Autodesk Inventor part; units mm, degrees
ref_plane "Work Plane4" through (-13.97, 12.7, 0) normal (0, 1, 0) x (1, 0, 0)
ref_plane "Work Plane5" through (-3.3455, -30.0155, 0) normal (0, 1, 0) x (-1, 0, 0)
ref_plane "YZ Plane" through (0, 0, 0) normal (1, 0, 0) x (0, 1, 0)
sketch "Sketch1" plane through (0, 0, 0) normal (0, 0, 1) x (1, 0, 0)
  line L0 (-13.97, -12.7) -> (13.97, -12.7)
  line L1 (13.97, -12.7) -> (13.97, 12.7)
  line L2 (13.97, 12.7) -> (-13.97, 12.7)
  line L3 (-13.97, 12.7) -> (-13.97, -12.7)
  line L4 (-13.97, -12.7) -> (13.97, 12.7) construction
  line L5 (13.97, -12.7) -> (-13.97, 12.7) construction
  arc A0 (-13.97, -12.7) -> (13.97, -12.7) centre (0, -12.7) ccw
  circle A1 centre (-3.3455, -12.7) radius 11.811
  line L6 (0, -12.7) -> (-13.97, -12.7)
  line L7 (0, -12.7) -> (-6.985, -12.7)
  circle A2 centre (-3.3455, -12.7) radius 17.3155
  arc A3 (-20.6609, -12.7) -> (-13.97, 12.7) centre (-56.001, 10.1906) ccw
  point P0 (0, 0)
  point P1 (-15.1565, -0.038)
  dimension "d0" = 27.94
  dimension "d1" = 25.4
  dimension "d2" = 23.622
sketch "Sketch5" plane through (0, 0, 0) normal (0, 0, 1) x (1, 0, 0)
  line L0 (0, 12.7) -> (0, 6.35)
  line L1 (0, 12.7) -> (0, 9.525)
  line L2 (5.715, 7.3025) -> (-5.715, 7.3025)
  line L3 (-5.715, 7.3025) -> (-5.715, 11.7475)
  line L4 (-5.715, 11.7475) -> (5.715, 11.7475)
  line L5 (5.715, 11.7475) -> (5.715, 7.3025)
  line L6 (5.715, 7.3025) -> (-5.715, 11.7475) construction
  line L7 (-5.715, 7.3025) -> (5.715, 11.7475) construction
  line L8 (5.715, 11.7475) -> (3.175, 11.7475)
  line L9 (3.175, 11.7475) -> (3.175, 10.7597)
  line L10 (3.175, 10.7597) -> (5.715, 10.7597)
  line L11 (5.715, 10.7597) -> (5.715, 11.7475)
  line L12 (-5.715, 11.7475) -> (-3.2581, 11.7475)
  line L13 (-3.2581, 11.7475) -> (-3.2581, 10.792)
  line L14 (-3.2581, 10.792) -> (-5.715, 10.792)
  line L15 (-5.715, 10.792) -> (-5.715, 11.7475)
  line L16 (5.715, 9.525) -> (3.175, 7.3025)
  line L17 (-5.715, 9.525) -> (-3.175, 7.3025)
  point P0 (0, 0)
  point P1 (5.715, 10.7597)
  point P2 (-3.2581, 11.7475)
  point P3 (-5.715, 10.792)
  dimension "d5" = 4.445
  dimension "d6" = 11.43
  dimension "d7" = 2.54
ref_plane "Work Plane4" through (-13.97, 12.7, 0) normal (0, 1, 0) x (1, 0, 0)
sketch "Sketch6" plane through (-13.97, 12.7, 0) normal (0, 1, 0) x (1, 0, 0)
  circle A0 centre (13.5492, -9.5343) radius 2.54
  dimension "d19" = 5.08
extrude "Extrusion7" add sketch "Sketch1" along normal blind 19.05 contours A1 A0 A2 A3 L3 | L3 A2 L0 A1 | A1 L0 A0 | A2 A3 L3 | L3 A3 L2 L1 A2 | A3 A2 picked at (12.0052, -13.7923)
extrude "Extrusion8" cut sketch "Sketch5" along normal blind 20.32 contours L4 L9 L10 L5 L16 L2 L0 | L0 L2 L17 L3 L14 L13 L4
extrude "Extrusion9" cut sketch "Sketch6" against normal blind 15.24
fillet "Fillet1" radius 3.175 1 edges at (-15.1565, -0.038, 9.525)
sketch "Sketch10" plane through (-13.97, 12.7, 0) normal (0, 1, 0) x (1, 0, 0)
  line L0 (13.97, 0) -> (13.97, -20.32)
  line L1 (0.0748, -19.05) -> (0.0748, 0)
  line L2 (0.0748, -9.525) -> (27.94, -9.525)
  line L3 (27.94, 0) -> (27.94, -19.05)
  line L4 (3.9773, -13.335) -> (1.6913, -13.335)
  line L5 (1.6913, -13.335) -> (1.6913, -5.715)
  line L6 (1.6913, -5.715) -> (3.9773, -5.715)
  line L7 (3.9773, -5.715) -> (3.9773, -13.335)
  line L8 (3.9773, -13.335) -> (1.6913, -5.715) construction
  line L9 (1.6913, -13.335) -> (3.9773, -5.715) construction
  line L10 (23.9627, -13.335) -> (26.2487, -13.335)
  line L11 (26.2487, -13.335) -> (26.2487, -5.715)
  line L12 (26.2487, -5.715) -> (23.9627, -5.715)
  line L13 (23.9627, -5.715) -> (23.9627, -13.335)
  point P0 (2.8343, -9.525)
  dimension "d32" = 2.286
  dimension "d33" = 7.62
extrude "Extrusion10" cut sketch "Sketch10" against normal blind 2.54
ref_plane "Work Plane5" through (-3.3455, -30.0155, 0) normal (0, 1, 0) x (-1, 0, 0)
sketch "Sketch11" plane through (-3.3455, -30.0155, 0) normal (0, 1, 0) x (-1, 0, 0)
  line L0 (-0.1705, 0) -> (-0.1705, 19.05)
  circle A0 centre (-0.1705, 9.525) radius 2.54
  point P0 (-3.3455, 0)
  dimension "d36" = 5.08
extrude "Extrusion11" cut sketch "Sketch11" along normal blind 15.24
properties part number "MotorBearingHolder"
CAD build for the part. Positions are in the model's coordinates, mm. A direction names the side the tool comes from. Round coordinates to 2 decimals unless told otherwise and drop trailing zeros. Write each loop counter-clockwise with the first axis right and the second up, starting at its lowest first coordinate (ties: lowest second). Pieces come first, ordered by that corner, then holes.
(1) Slice it at D-D, the plane z = 14. Count the separate pieces of the cut face and the enclosed holes in it, and give its area (3 significant figures).
(2) Mould opens along Z. For faces 4 (the face through (9.993, 11, 9)), 5 (the face through (-14.03, 6.84, 9.39)), 6 (the face through (11, 11, 5.715)) say: pulls with the +Z half, pulls with the -Z half, needs draft (parallel to the pull), parting line crosses it, or undercut.
(3) Slice it at B-B, the plane x = -9.5. Write the cut outline in (y, z).
(4) Probe line 1 along Y through (x, z) = (5, 12.75); line 2 along Y through (x, z) = (2.5, 9.75); line 3 along X through (y, z) = (-12.7, 7.5). List the from-to ranges inside material, lowest first.
(5) Slice it at C-C, the plane x = -4. Write the cut outline in (y, z), and give its area (3 significant figures).
(6) Drop flat-ended pins along their axis: P1, Ø1.3, axis at y = 11.5, z = 11, coming from the -X side; P2, Ø2, axis at x = -6, y = -22, coming from the +Z side; P3, Ø1.8, axis at x = 11, z = 11, coming from the +Y side; P4, Ø3, axis at x = -0.5, z = 12, coming from the -Y side. Give the stop position or say it passes through.
(7) 3-axis set-ups, long thin cutter, end or side, ignore diameter. For faces 1 (the face through (-12.279, 11, 10)), 2 (the face through (-4, 10.792, 9)), 3 (the face through (13.97, 0, 9)): which of +Z, -Z, +X, -X, +Y, -Y reach the whole face in a straight line?
(8) Slice it at A-A, the plane y = -21. Write the cut outline in (x, z).
From the geometry:
1. separate pieces: 1
1. enclosed holes: 2
1. area: 769 mm2
2. face 4: undercut
2. face 5: needs draft
2. face 6: undercut
3. outline: (-28.88, 0) - (-22.78, 0) - (-22.78, 19.05) - (-28.88, 19.05) - close; (-2.62, 0) - (12.7, 0) - (12.7, 19.05) - (-2.62, 19.05) - close
4. line 1: y = -27.87 to -21.06, -4.34 to 8.9, 10.76 to 12.7
4. line 2: y = -29 to -22.96, -2.44 to 7.3, 11.75 to 12.7
4. line 3: x = -20.66 to -15.16, 8.47 to 13.97
5. outline: (-30, 0) - (-24.49, 0) - (-24.49, 7.12) - (-30, 7.12) - close; (-30, 11.93) - (-24.49, 11.93) - (-24.49, 19.05) - (-30, 19.05) - close; (-0.91, 0) - (8.02, 0) - (8.02, 19.05) - (-0.91, 19.05) - close; (10.79, 0) - (12.7, 0) - (12.7, 19.05) - (10.79, 19.05) - close
5. area: 285 mm2
6. P1: stops at x = -13.94
6. P2: passes through
6. P3: stops at y = 10.16
6. P4: stops at y = -29.96
7. face 1: +Y
7. face 2: +Z, -Z
7. face 3: +Z, -Z, +X, +Y, -Y
8. outline: (-18.54, 0) - (-11.75, 0) - (-11.75, 19.05) - (-18.54, 19.05) - close; (5.06, 0) - (11.85, 0) - (11.85, 19.05) - (5.06, 19.05) - close
